Read the model definition and answer for the solid it produces. Units are mm, in the model's axes. Coordinates: 2 decimals unless noted, no trailing zeros. Order: outer loops, then holes, each group sorted by start corner. A loop starts at its lowest first (then second) coordinate and runs counter-clockwise, first axis right, second up. Notation, with made-up numbers: (-8.75, 47) -> (38.25, 47) arc R31 cw to (38.25, 82) -> close; hole circle Ø10 at (5.25, 10.5). An arc over 180 degrees is marked (long way). Answer in a Markdown table with one row per item.
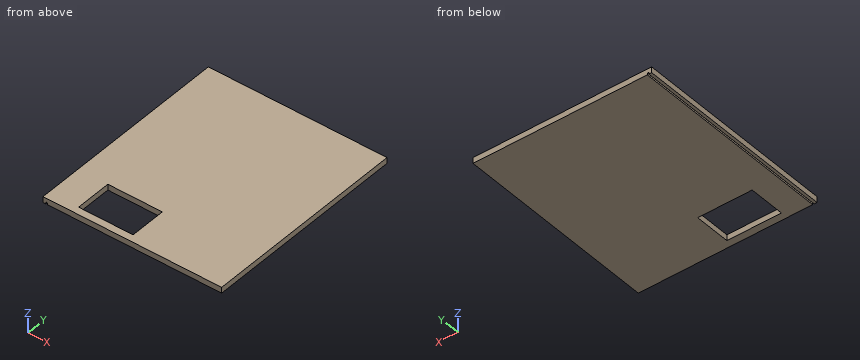
from build123d import *

# Parameters (mm, degrees)
F0_W     = 492
F0_H     = 566
F1_DEPTH = 16
F2_W     = 150
F2_H     = 100
F3_DEPTH = 16.001
F4_W     = 4
F4_H     = 5
F5_DEPTH = 566.001


with BuildPart() as f1:
    # F0 (on Top) → F1 (new body)
    with BuildSketch(Plane.XY):
        Rectangle(F0_W, F0_H)
    extrude(amount=F1_DEPTH)

    # F2 (on face) → F3 (cut, through all)
    with BuildSketch(Plane.XY.offset(16)):
        with Locations((-89, -213)):
            Rectangle(F2_W, F2_H)
    extrude(amount=-F3_DEPTH, mode=Mode.SUBTRACT)

    # F4 (on face) → F5 (cut, through all)
    with BuildSketch(Plane(origin=(0, 283, 0), x_dir=(-1, 0, 0), z_dir=(0, 1, 0))):
        with Locations((236, 2.5)):
            Rectangle(F4_W, F4_H)
    extrude(amount=-F5_DEPTH, mode=Mode.SUBTRACT)


solid = f1.part
Q1. The part is cut by section B-B (x = -54). Write down the section's boundary in (y, z), then the cut area to 3 significant figures.
Outcome:
| item | result |
|---|---|
| outline | (-283, 0) -> (-263, 0) -> (-263, 16) -> (-283, 16) -> close; (-163, 0) -> (283, 0) -> (283, 16) -> (-163, 16) -> close |
| area | 7,460 mm² |
Q2. The part is cut by section C-C (z = 9). Write down the section's boundary in (x, y), then the cut area to 3 significant figures.
Outcome:
| item | result |
|---|---|
| outline | (-246, -283) -> (246, -283) -> (246, 283) -> (-246, 283) -> close; hole (-164, -263) -> (-14, -263) -> (-14, -163) -> (-164, -163) -> close |
| area | 263,000 mm² |
Q3. Given pin 1 (1.2 mm diameter, centred on x = -235.5, y = -73, fed in from -Z), flat-ended and moving along its own axis, determine where the tip first touches the part or whether it passes through.
Outcome:
| item | result |
|---|---|
| pin 1 | z = 5 |
Q4. Consider line 1 (X direction, y = 156.5, z = 3.5); line 2 (Y direction, x = -53, z = 2.5); line 3 (X direction, y = -239.5, z = 14.25). Determine where each line is inside the solid, lowest interval first.
Outcome:
| item | result |
|---|---|
| line 1 | -246 to -238, -234 to 246 |
| line 2 | -283 to -263, -163 to 283 |
| line 3 | -246 to -164, -14 to 246 |
Q5. The part is cut by section A-A (y = -196). Write down the section's boundary in (x, z), then the cut area to 3 significant figures.
Outcome:
| item | result |
|---|---|
| outline | (-246, 0) -> (-238, 0) -> (-238, 5) -> (-234, 5) -> (-234, 0) -> (-164, 0) -> (-164, 16) -> (-246, 16) -> close; (-14, 0) -> (246, 0) -> (246, 16) -> (-14, 16) -> close |
| area | 5,450 mm² |
